Part print with two shaded views. Sizes in mm from the minimum x, y, z corner. A direction names the side the tool comes from. Round coordinates to 2 decimals unless told otherwise and drop trailing zeros. Write each loop counter-clockwise with the first axis right and the second up, starting at its lowest first coordinate (ties: lowest second). Pieces come first, ordered by that corner, then holes. Notation, with made-up numbers: (56.5, 67) - (97.5, 67) arc R21 ccw to (97.5, 71) - close; hole circle Ø2 at (36, 49). An arc over 180 degrees is marked (long way). Use one line per item in the form item = value. Start each with the question number.
Item 1: Band-saw the part on A-A, the plane x = 4.5. List the corners of the cut face in (y, z).
Item 2: Drill centre lines: L1, parallel to Y at x = 9.75, z = 4.35; L2, parallel to Z at x = 17, y = 12; L3, parallel to Y at x = 10, z = 2 (1 decimal). Where is each one in solid material? Low to high.
Item 3: Band-saw the part on D-D, the plane x = 10.5. List the corners of the cut face in (y, z).
Item 4: Band-saw the part on C-C, the plane z = 3.8. List the corners of the cut face in (x, y).
Item 5: Pin check, flat tips, straight feed: pin 1 (1.5 mm diameter, centred on y = 32.5, z = 3, fed in from -X); pin 2 (2.5 mm diameter, centred on x = 7, z = 3.5, fed in from +Y); pin 3 (7.5 mm diameter, centred on x = 8.5, y = 13, fed in from +Z); pin 4 (1 mm diameter, centred on x = 4.5, y = 10.5, fed in from +Z). Stop position of each tip, or through.
Item 6: Tool access for the marked faces 1 and 2: list every direction of +Z, -Z, +X, -X, +Y, -Y with a clear straight run to the whole face (end or side of a thin tool).
Item 7: Band-saw the part on B-B, the plane y = 10.5. List the corners of the cut face in (x, z) (1 decimal).
Item 8: Pull direction Y, two halves, no side cores. Call the marked faces 3, 4 and 5: +Y half, -Y half, draft (parallel to the pull), parting line (faces both ways), or undercut.
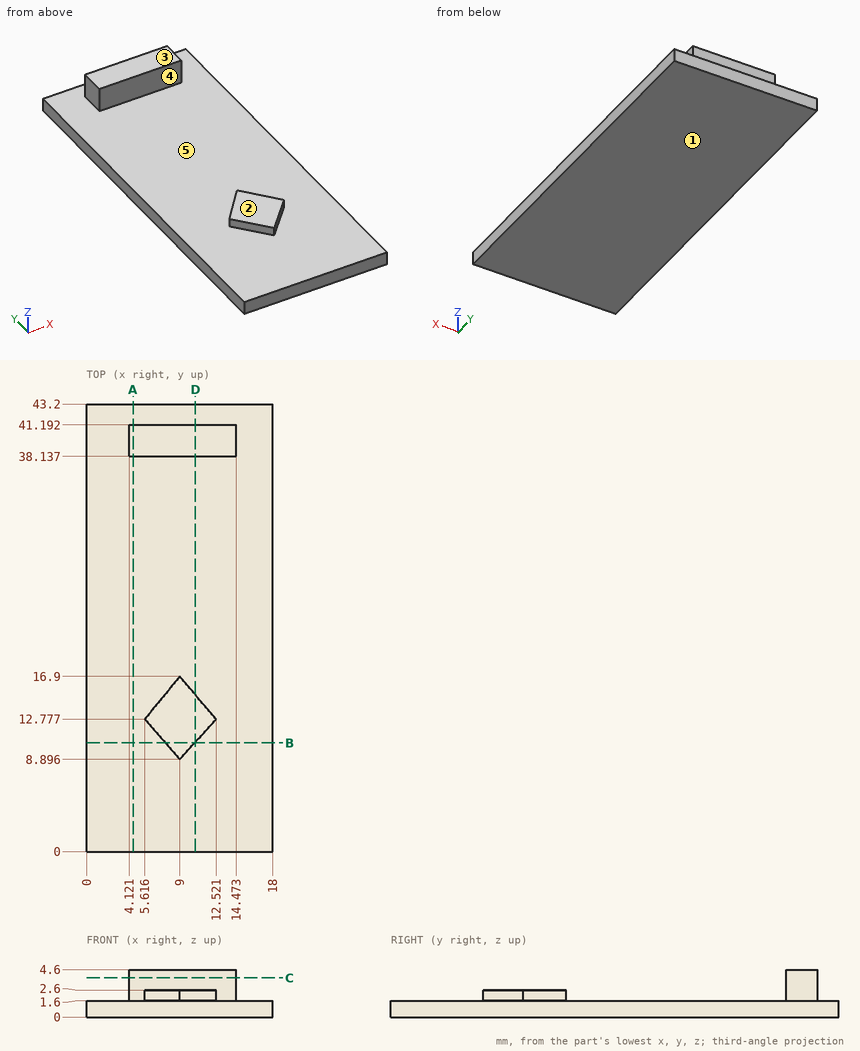
Determined:
q1.outline = (0, 0) - (43.2, 0) - (43.2, 1.6) - (41.19, 1.6) - (41.19, 4.6) - (38.14, 4.6) - (38.14, 1.6) - (0, 1.6) - close
q2.L1 = 38.14 to 41.19
q2.L2 = 0 to 1.6
q2.L3 = 10 to 15.7, 38.1 to 41.2
q3.outline = (0, 0) - (43.2, 0) - (43.2, 1.6) - (41.19, 1.6) - (41.19, 4.6) - (38.14, 4.6) - (38.14, 1.6) - (15.14, 1.6) - (15.14, 2.6) - (10.55, 2.6) - (10.55, 1.6) - (0, 1.6) - close
q4.outline = (4.12, 38.14) - (14.47, 38.14) - (14.47, 41.19) - (4.12, 41.19) - close
q5.pin_1 = through
q5.pin_2 = 41.19
q5.pin_3 = 2.6
q5.pin_4 = 1.6
q6.face_1 = -Z, +X, -X, +Y, -Y
q6.face_2 = +Z, +X, -X, -Y
q7.outline = (0, 0) - (18, 0) - (18, 1.6) - (10.5, 1.6) - (10.5, 2.6) - (7.6, 2.6) - (7.6, 1.6) - (0, 1.6) - close
q8.face_3 = draft
q8.face_4 = undercut
q8.face_5 = undercut
